```python
from build123d import *

# Parameters (mm, degrees)
CROQUIS1_R              = 1.5
SALIENTE_EXTRUIR1_DEPTH = 29


with BuildPart() as part:
    # Croquis1 → Saliente-Extruir1 (new, symmetric)
    with BuildSketch(Plane.XY):
        Polygon((4.618802154, 0), (2.309401077, 4), (-2.309401077, 4), (-4.618802154, 0), (-2.309401077, -4), (2.309401077, -4), align=None)
        with Locations(Location((0, 0, 0), (0, 0, 180))):
            Circle(CROQUIS1_R, mode=Mode.SUBTRACT)
    extrude(amount=SALIENTE_EXTRUIR1_DEPTH, both=True)


solid = part.part
```
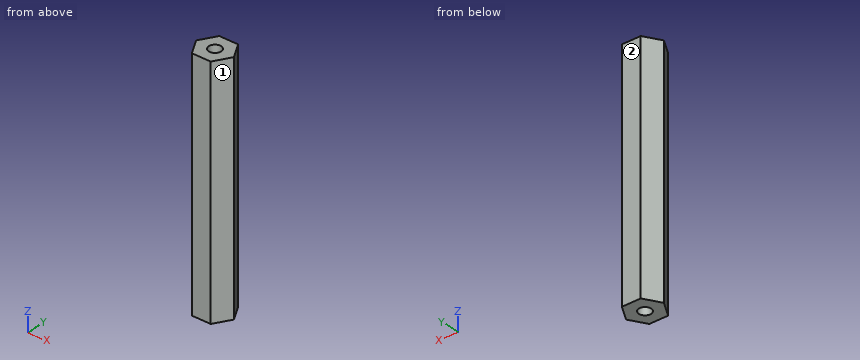
Build history of the part. All positions in model axes, mm. Face numbers are marked on the shaded views. Round coordinates to 2 decimals unless told otherwise and drop trailing zeros. Order: outer loops, then holes, each group sorted by start corner. A loop starts at its lowest first (then second) coordinate and runs counter-clockwise, first axis right, second up. Notation, with made-up numbers: (-25, -0.5) - (9, -0.5) arc R33 cw to (9, 31.5) - close; hole circle Ø6 at (3.5, -15). An arc over 180 degrees is marked (long way). Use a Markdown table: item, result.
1) Flat gauge pins, fed straight in: pin 1 Ø4 at (y, z) = (1, 16) entering from -X; pin 2 Ø1.5 at (x, z) = (3.5, 15.5) entering from +Y. Where does each tip first touch, or does it go through?
Recorded:
| item | result |
|---|---|
| pin 1 | stops at x = -4.62 |
| pin 2 | stops at y = 3.24 |
2) Saw through at B-B on z = 15. Write the cut outline in (x, y).
Recorded:
| item | result |
|---|---|
| outline | (-4.62, 0) - (-2.31, -4) - (2.31, -4) - (4.62, 0) - (2.31, 4) - (-2.31, 4) - close; hole circle Ø3 at (0, 0) |
3) Saw through at A-A on x = 0. Write the cut outline in (y, z).
Recorded:
| item | result |
|---|---|
| outline | (-4, -29) - (-1.5, -29) - (-1.5, 29) - (-4, 29) - close; (1.5, -29) - (4, -29) - (4, 29) - (1.5, 29) - close |
4) Saw through at C-C on x = 3.25. Write the cut outline in (y, z), and give its area (3 significant figures).
Recorded:
| item | result |
|---|---|
| outline | (-2.37, -29) - (2.37, -29) - (2.37, 29) - (-2.37, 29) - close |
| area | 275 mm² |
5) Pull direction Y, two halves, no side cores. Call the marked faces 1 and 2: pulls with the +Y half, pulls with the -Y half, needs draft (parallel to the pull), parting line crosses it, or undercut.
Recorded:
| item | result |
|---|---|
| face 1 | pulls with the -Y half |
| face 2 | pulls with the +Y half |
6) Wall check: L1, parallel to Y at x = 0, z = 13; L2, parallel to Y at x = 3.75, z = -20; L3, parallel to X at y = 0.25, z = -9. Give the ranges that are in metal, low to high.
Recorded:
| item | result |
|---|---|
| L1 | y = -4 to -1.5, 1.5 to 4 |
| L2 | y = -1.5 to 1.5 |
| L3 | x = -4.47 to -1.48, 1.48 to 4.47 |
